Autodesk Inventor part; units mm, degrees
ref_plane "YZ Plane" through (0, 0, 0) normal (1, 0, 0) x (0, 1, 0)
ref_plane "XY Plane" through (0, 0, 0) normal (0, 0, 1) x (1, 0, 0)
sketch "Sketch1" plane through (0, 0, 0) normal (0, 0, 1) x (1, 0, 0)
  circle A0 centre (84.114, 58.3351) radius 15.24
  line L0 (84.114, 61.4651) -> (84.114, 53.9668)
  line L1 (87.092, 58.3351) -> (81.5348, 58.3351)
  point P0 (0, 0)
  dimension "d0" = 30.48
extrude "Extrusion1" add sketch "Sketch1" along normal blind 40.64
sketch "Sketch2" plane through (84.114, 58.3351, 40.64) normal (0, 0, 1) x (1, 0, 0)
  circle A0 centre (0, 0) radius 11.8999
  circle A1 centre (0, 0) radius 0.381
  point P0 (-84.114, -58.3351)
  dimension "d3" = 23.7998
  dimension "d62" = 0.762
extrude "Extrusion2" add sketch "Sketch2" along normal blind 6.35 contours A0 | A1
chamfer "Chamfer1" distance 0.508 angle 45 1 edges at (72.2141, 58.3351, 46.99)
chamfer "Chamfer2" distance 1.016 angle 45 1 edges at (68.874, 58.3351, 40.64)
thread "Thread2"
sketch "Sketch4" plane through (84.114, 58.3351, 0) normal (0, 0, -1) x (-1, 0, 0)
  circle A0 centre (0, 0) radius 11.8999
  point P0 (84.114, -58.3351)
hole "Hole1" at (84.114, 58.3351, 0) direction (0, 0, 1) diameter 15.24 depth 41.91 tip angle 120
chamfer "Chamfer3" distance 1.016 angle 45 1 edges at (68.874, 58.3351, 0)
sketch "Sketch9" plane through (84.114, 58.3351, 46.99) normal (0, 0, 1) x (1, 0, 0)
  point P0 (0, 0)
hole "Hole3" at (84.114, 58.3351, 46.99) direction (0, 0, 1) diameter 0.762 depth 41.91 tip angle 120
sketch "Sketch10" plane through (84.114, 58.3351, 46.99) normal (0, 0, 1) x (1, 0, 0)
  circle A0 centre (0, 0) radius 0.381
  point P0 (-84.114, -58.3351)
  dimension "d63" = 0.762
extrude "Extrusion6" cut sketch "Sketch10" against normal blind 7.62
ref_plane "Work Plane11" through (84.114, 43.0951, 0) normal (0, 1, 0) x (-1, 0, 0)
sketch "Sketch12" plane through (84.114, 43.0951, 0) normal (0, 1, 0) x (-1, 0, 0)
  circle A0 centre (0, 36.83) radius 1.4224
  circle A1 centre (0, 3.81) radius 1.4224
  point P0 (84.114, 0)
  dimension "d68" = 2.8448
  dimension "d69" = 2.8448
  dimension "d71" = 33.02
sketch "Sketch19" plane through (84.114, 43.0951, 0) normal (0, 1, 0) x (-1, 0, 0)
  point P0 (84.114, 0)
sketch "Sketch20" plane through (84.114, 43.0951, 0) normal (0, 1, 0) x (-1, 0, 0)
  circle A0 centre (-0.009, 36.83) radius 1.27
  circle A1 centre (-0.009, 3.81) radius 1.27
  line L0 (-11.3919, 46.99) -> (11.3919, 46.99)
  point P0 (84.114, 0)
  dimension "d78" = 2.54
  dimension "d79" = 2.54
  dimension "d80" = 10.16
  dimension "d81" = 33.02
extrude "Extrusion9" cut sketch "Sketch20" along normal blind 8.89
sketch "Sketch21" plane through (84.114, 43.0951, 0) normal (0, 1, 0) x (-1, 0, 0)
  point P0 (84.114, 0)
sketch "Sketch22" plane through (84.114, 43.0951, 0) normal (0, 1, 0) x (-1, 0, 0)
  point P0 (84.114, 0)
  point P1 (27.3328, 48.7683)
  point P2 (26.9749, -2.1467)
  point P3 (-27.3472, -1.8634)
  point P4 (-26.971, 48.9999)
ref_plane "Work Plane17" through (57.1391, 43.0951, -2.1467) normal (-0.866, 0.5, -0.0061) x (-0.007, 0, 1)
sketch "Sketch23" plane through (57.1391, 43.0951, -2.1467) normal (-0.866, 0.5, -0.0061) x (-0.007, 0, 1)
  circle A0 centre (38.7859, 26.8321) radius 1.4224
  circle A1 centre (5.7659, 26.8321) radius 1.4224
  ellipse E0 centre (48.9459, 26.858) end of major axis (48.9058, 38.2499) minor radius 0.0694
  point P0 (2.5484, -65.8828)
  dimension "d88" = 2.8448
  dimension "d89" = 2.8448
  dimension "d90" = 10.16
  dimension "d91" = 33.02
extrude "Extrusion10" cut sketch "Sketch23" against normal blind 8.89 contours A0 | A1
ref_plane "Work Plane18" through (111.085, 43.0951, 48.9999) normal (0.866, 0.5, 0.0064) x (0.0074, 0, -1)
sketch "Sketch24" plane through (111.085, 43.0951, 48.9999) normal (0.866, 0.5, 0.0064) x (0.0074, 0, -1)
  circle A0 centre (11.9704, 26.7143) radius 1.4224
  circle A1 centre (44.9904, 26.7143) radius 1.4224
  ellipse E0 centre (1.8104, 26.6908) end of major axis (1.7683, 38.0826) minor radius 0.073
  point P0 (48.177, 18.4007)
  dimension "d95" = 2.8448
  dimension "d96" = 2.8448
  dimension "d97" = 10.16
  dimension "d98" = 33.02
extrude "Extrusion11" cut sketch "Sketch24" against normal blind 8.89 contours A0 | A1
thread "Thread3"
properties part number "laserfocus"
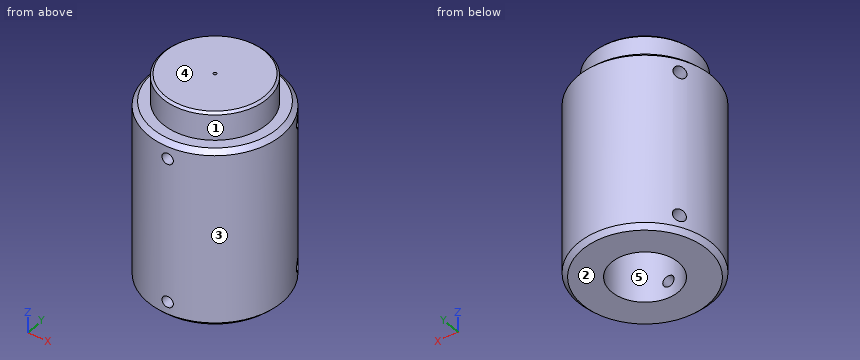
Input: part model. Units: mm. Frame: model coordinates. Face numbers are marked on the shaded views. A direction names the side the tool comes from. Give positions to 0.01 mm unless a question says otherwise; leave off trailing zeros. Write each loop counter-clockwise with the first axis right and the second up, starting at its lowest first coordinate (ties: lowest second). Pieces come first, ordered by that corner, then holes. Notation, with made-up numbers: (16, -8.75) -> (40, -8.75) arc R13 cw to (40, 12.25) -> close; hole circle Ø4 at (59, 41). An arc over 180 degrees is marked (long way). Use one line per item in the form item = value. Start each with the question number.
1) Draft query along X for the marked faces 3, 4 and 5. Return one class per face: pulls with the +X half, pulls with the -X half, needs draft (parallel to the pull), parting line crosses it, or undercut.
2) Ray query, probe 1 along Y at (x, z) = (84, 11); probe 2 along Z at (x, y) = (85, 47.5); probe 3 along Y at (x, z) = (80, 3.5). Return the intervals inside material, ascending. Write a range as from..to.
3) Set-up query: the marked faces 1 and 2. Return all of +Z, -Z, +X, -X, +Y, -Y with unobstructed straight access to the full face (end or side cutting, diameter ignored); none if empty.
4) Pin query (flat end, axial travel): pin 1 (3 mm diameter, centred on x = 84.123, z = 36.83, fed in from -Y); pin 2 (3 mm diameter, centred on x = 79.5, y = 56.5, fed in from -Z); pin 3 (12 mm diameter, centred on x = 84.11, y = 58.34, fed in from -Z); pin 4 (4 mm diameter, centred on x = 93, z = 12, fed in from -Y). Return the tip coordinate at first contact, or that it passes through.
5) Section query B-B on z = 13. Return the cut outline in (x, y), then the cut area to 3 significant figures.
6) Section query A-A on z = 36.83. Count the separate pieces of the cut face and the enclosed holes in it, then the cut area to 3 significant figures.
Outcome:
q1.face_3 = parting line crosses it
q1.face_4 = needs draft
q1.face_5 = undercut
q2.probe_1 = 43.1..50.72, 65.95..73.57
q2.probe_2 = 0..2.89, 4.73..35.91, 37.75..46.99
q2.probe_3 = 43.66..51.92, 64.75..73.01
q3.face_1 = +Z
q3.face_2 = -Z, +X, -X, +Y, -Y
q4.pin_1 = 43.1
q4.pin_2 = 42.58
q4.pin_3 = 42.84
q4.pin_4 = 44.74
q5.outline = circle Ø30.48 at (84.11, 58.34); hole circle Ø15.24 at (84.11, 58.34)
q5.area = 547 mm^2
q6.separate_pieces = 3
q6.enclosed_holes = 0
q6.area = 484 mm^2
